CAD build for the part. Positions are in the model's coordinates, mm. A direction names the side the tool comes from. Give positions to 0.01 mm unless a question says otherwise; leave off trailing zeros. Order: outer loops, then holes, each group sorted by start corner. A loop starts at its lowest first (then second) coordinate and runs counter-clockwise, first axis right, second up.
Item 1: Two-plate mould, pull along Y, no slides. Class faces 4 (the cylindrical face through (-18.783, 36.934, -48.335)), 5 (the flat face through (-18.78, 61.52, -22.16)), 6 (the flat face through (-19, -56, -30.197)): released by +Y, released by -Y, zero draft, split by the parting line, or undercut.
Item 2: Band-saw the part on D-D on z = -27.5. Give the cut face in (x, y).
Item 3: Band-saw the part on A-A on z = -40. Give the cut face in (x, y), plus the area to 3 significant figures.
Item 4: Band-saw the part on C-C on y = 30. Give the cut face in (x, z).
Item 5: Flat gauge pins, fed straight in: P1, Ø5, axis at x = -31.5, y = -18, coming from the -Z side; P2, Ø8, axis at x = -31.5, z = 36.5, coming from the +Y side; P3, Ø4, axis at x = -16, z = 37, coming from the -Y side; P4, Ø8, axis at y = 35.5, z = 11, coming from the +X side. Where does each tip first touch, or does it go through?
Item 6: Wall check: L1, parallel to Z at x = -16, y = -50.5; L2, parallel to Y at x = -25.5, z = -40.5; L3, parallel to Z at x = -5, y = 15. Give the ranges that are in metal, low to high.
Item 7: Which spindle directions (+Z, -Z, +X, -X, +Y, -Y) get a long thin tool onto all of the face, cutting with end or side? Do faces 1 (the flat face through (-19, 56, -32.977)), 2 (the flat face through (0, 10, 3)), 3 (the flat face through (-19, -57, 0)). Say none if no direction does.
Item 8: Band-saw the part on B-B on x = -2.5. Give the cut face in (y, z).
```python
from build123d import *

# Parameters (mm, degrees)
F1_DEPTH = 38.1


with BuildPart() as f1:
    # F0 (on Right) → F1 (new body)
    with BuildSketch(Plane.YZ):
        with BuildLine():
            Line((44.800351, 52.902363), (-25.254121, 52.902363))
            Line((-25.254121, 52.902363), (-43.48034, 0))
            Line((-43.48034, 0), (-71.900882, 0))
            Line((-71.900882, 0), (-68.193853, -30.196825))
            Line((-68.193853, -30.196825), (-43.48034, -30.196825))
            ThreePointArc((-43.48034, -30.196825), (-27.571015, -45.091976), (-11.661689, -30.196825))
            Line((-11.661689, -30.196825), (23.863986, -30.196825))
            ThreePointArc((23.863986, -30.196825), (37.289157, -48.372257), (53.829122, -32.977093))
            Line((53.829122, -32.977093), (59.080742, -32.977093))
            Line((59.080742, -32.977093), (64.023443, -11.043851))
            Line((64.023443, -11.043851), (44.800351, 52.902363))
        make_face()
    extrude(amount=-F1_DEPTH)


solid = f1.part
```
The answers:
1. face 4: undercut
1. face 5: released by +Y
1. face 6: zero draft
2. outline: (-38.1, -68.52) - (0, -68.52) - (0, 60.32) - (-38.1, 60.32) - close
3. outline: (-38.1, -39.25) - (0, -39.25) - (0, -15.89) - (-38.1, -15.89) - close; (-38.1, 25.11) - (0, 25.11) - (0, 52.27) - (-38.1, 52.27) - close
3. area: 1,920 mm2
4. outline: (-38.1, -45.7) - (0, -45.7) - (0, 52.9) - (-38.1, 52.9) - close
5. P1: stops at z = -43.44
5. P2: stops at y = 50.93
5. P3: stops at y = -31.42
5. P4: stops at x = 0
6. L1: z = -30.2 to 0
6. L2: y = -38.77 to -16.38, 25.37 to 52.01
6. L3: z = -30.2 to 52.9
7. face 1: -Z, +X, -X, +Y
7. face 2: +Z, -Z, +X, +Y, -Y
7. face 3: +Z, +X, -X, -Y
8. outline: (-71.9, 0) - (-68.19, -30.2) - (-43.48, -30.2) arc R15.94 ccw to (-11.66, -30.2) - (23.86, -30.2) arc R15.14 ccw (long way) to (53.83, -32.98) - (59.08, -32.98) - (64.02, -11.04) - (44.8, 52.9) - (-25.25, 52.9) - (-43.48, 0) - close
